Could you check a few things on this model? Use its own coordinates, in mm. A direction names the side the tool comes from. Coordinates: 2 decimals unless noted, no trailing zeros. Loops run counter-clockwise (first coordinate to the right, second up) from the corner with the lowest first, then second, coordinate; pieces in that order, holes last.
1) Thinking about a two-plate mould opening in Y: for faces 1 (the face through (0, 0, -15)), 2 (the face through (-1.25, 0, 2)), 3 (the face through (-0.596, 2.685, 1.479)), which applies, released by +Y, released by -Y, zero draft, split by the parting line, or undercut?
2) Imagine slicing it at B-B on x = 0.9. Please give me the cut outline in (y, z), plus the area to 3 significant figures.
3) Imagine slicing it at A-A on y = 0. Please give me the cut outline in (x, z).
4) Imagine slicing it at D-D on y = 2.1. Please give me the cut outline in (x, z), plus the area to 3 significant figures.
5) If I drill on line 1 along Z through (x, y) = (-0.4, -1.65); line 2 along X through (y, z) = (0.4, -1); line 3 along Z through (x, y) = (0.6, 0.8), over which ranges is the centre line in solid material (lowest first)?
6) Imagine slicing it at C-C on z = -13. Please give me the cut outline in (x, y), plus the area to 3 significant figures.
7) Will this pin go through, and if not, where does the flat tip stop? P1, Ø3, axis at x = 0, y = 0.5, coming from the +Z side.
8) For faces 4 (the face through (0.6, 1.3, 3)), 5 (the face through (-1.5, 0.07, -7.4)), 6 (the face through (0.616, 1.088, 2.359)), which set-ups out of +Z, -Z, +X, -X, +Y, -Y let a thin tool reach every point of the face, with its end or its side?
Autodesk Inventor part; units mm, degrees
ref_plane "YZ Plane" through (0, 0, 0) normal (1, 0, 0) x (0, 1, 0)
ref_plane "XZ Plane" through (0, 0, 0) normal (0, 1, 0) x (-1, 0, 0)
ref_plane "XY Plane" through (0, 0, 0) normal (0, 0, 1) x (1, 0, 0)
sketch "スケッチ1" plane through (0, 0, 0) normal (0, 0, 1) x (1, 0, 0)
  circle A0 centre (0, 0) radius 1.5
  dimension "d0" = 3
extrude "押し出し1" add sketch "スケッチ1" against normal blind 15
sketch "スケッチ2" plane through (0, 0, 0) normal (0, 0, 1) x (1, 0, 0)
  circle A0 centre (0, 0) radius 2.75
  dimension "d3" = 5.5
extrude "押し出し2" add sketch "スケッチ2" along normal blind 3
sketch "スケッチ3" plane through (0, 0, 3) normal (0, 0, 1) x (1, 0, 0)
  line L0 (0, 1.4434) -> (1.25, 0.7217)
  line L1 (1.25, 0.7217) -> (1.25, -0.7217)
  line L2 (1.25, -0.7217) -> (0, -1.4434)
  line L3 (0, -1.4434) -> (-1.25, -0.7217)
  line L4 (-1.25, -0.7217) -> (-1.25, 0.7217)
  line L5 (-1.25, 0.7217) -> (0, 1.4434)
  point P0 (0, 0)
  point P1 (0, 0)
  dimension "d6" = 2.5
extrude "押し出し3" cut sketch "スケッチ3" against normal blind 1.3
thread "ねじ1"
properties part number "M3キャップボルト 15" material "鋼、高強度、低合金"
Filled in:
1. face 1: zero draft
1. face 2: undercut
1. face 3: split by the parting line
2. outline: (-2.6, 0) - (-1.2, 0) - (-1.2, -15) - (1.2, -15) - (1.2, 0) - (2.6, 0) - (2.6, 3) - (0.92, 3) - (0.92, 1.7) - (-0.92, 1.7) - (-0.92, 3) - (-2.6, 3) - close
2. area: 49.2 mm2
3. outline: (-2.75, 0) - (-1.5, 0) - (-1.5, -15) - (1.5, -15) - (1.5, 0) - (2.75, 0) - (2.75, 3) - (1.25, 3) - (1.25, 1.7) - (-1.25, 1.7) - (-1.25, 3) - (-2.75, 3) - close
4. outline: (-1.78, 0) - (1.78, 0) - (1.78, 3) - (-1.78, 3) - close
4. area: 10.7 mm2
5. line 1: z = 0 to 3
5. line 2: x = -1.45 to 1.45
5. line 3: z = -15 to 1.7
6. outline: circle Ø3 at (0, 0)
6. area: 7.07 mm2
7. P1: stops at z = 3
8. face 4: +Z, +X, -X, +Y, -Y
8. face 5: -Z
8. face 6: +Z
